For this review, use the dimensioned drawing (mm, ordinates from the lowest corner) and the shaded views. Coordinates: 2 decimals unless noted, no trailing zeros. Order: outer loops, then holes, each group sorted by start corner. A loop starts at its lowest first (then second) coordinate and runs counter-clockwise, first axis right, second up. Notation, with made-up numbers: M 44,11.5 L 102,11.5 A10 ccw 102,29.5 Z; hole C 33,47 d3. An arc over 180 degrees is marked long. Answer as CSV lines item,"result". Start each with the question number.
Q1. The part is to be moulded in two halves that separate along X. For the marked faces 1, 2 and 3, say which applies: +X half, -X half, draft (parallel to the pull), parting line (faces both ways), or undercut.
Q2. Consider section A-A on z = 6.35. Write out the cut boundary in (x, y).
Q3. Wall thickness on L1, parallel to X at y = 1.25, z = 6.25; L2, parallel to Z at x = 34, y = 1 (1 decimal); L3, parallel to X at y = 0.5, z = 3.75 (1 decimal): over which ranges is each line inside the solid? List them lowest first. Write a range as [from, to].
Q4. Consider section B-B on y = 3.75. Write out the cut boundary in (x, z).
Q5. Consider section C-C on x = 34.5. Write out the cut boundary in (y, z).
Q6. Consider section D-D on z = 10.25. Write out the cut boundary in (x, y), and give its area (3 significant figures).
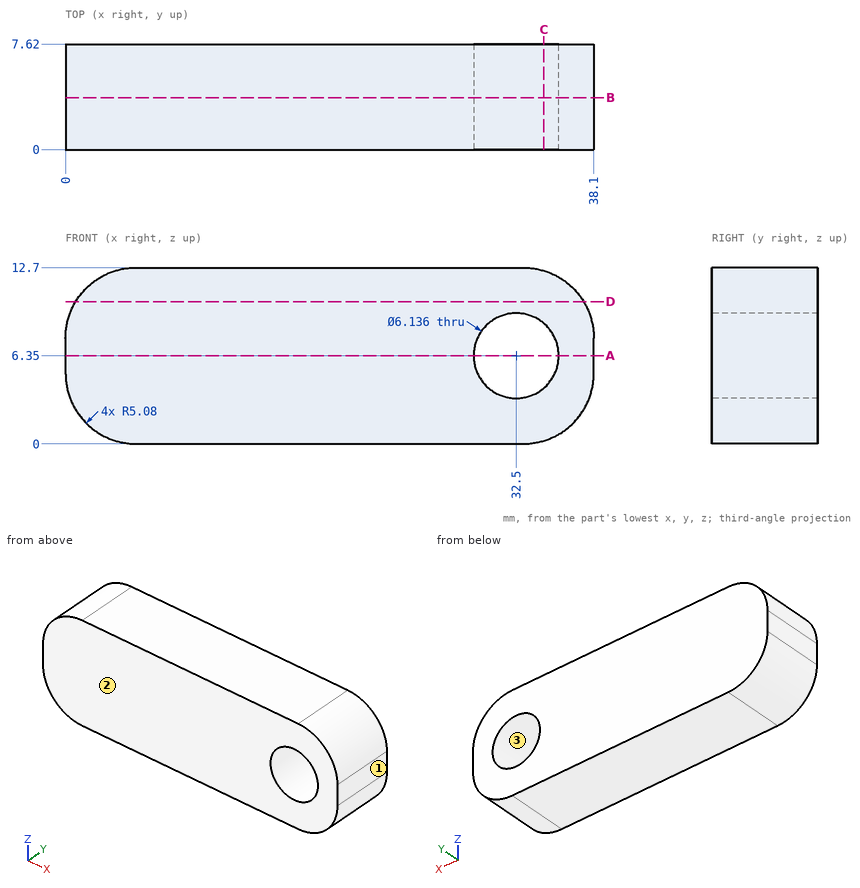
Evaluation:
1,face 1,"+X half"
1,face 2,"draft"
1,face 3,"undercut"
2,outline,"M 0,0 L 29.43,0 L 29.43,7.62 L 0,7.62 Z; M 35.57,0 L 38.1,0 L 38.1,7.62 L 35.57,7.62 Z"
3,L1,"x = [0, 29.43], [35.57, 38.1]"
3,L2,"z = [0.1, 3.7], [9, 12.6]"
3,L3,"x = [0.2, 30.9], [34.1, 37.9]"
4,outline,"M 0,5.08 A5.08 ccw 5.08,0 L 33.02,0 A5.08 ccw 38.1,5.08 L 38.1,7.62 A5.08 ccw 33.02,12.7 L 5.08,12.7 A5.08 ccw 0,7.62 Z; hole C 32.5,6.35 d6.14"
5,outline,"M 0,0.22 L 7.62,0.22 L 7.62,4.02 L 0,4.02 Z; M 0,8.68 L 7.62,8.68 L 7.62,12.48 L 0,12.48 Z"
6,outline,"M 0.73,0 L 37.37,0 L 37.37,7.62 L 0.73,7.62 Z"
6,area,"279 mm²"
